The model under review builds one solid part; all positions refer to its coordinate system, in mm. A direction names the side the tool comes from. Round coordinates to 2 decimals unless told otherwise and drop trailing zeros. Order: outer loops, then holes, each group sorted by start corner. A loop starts at its lowest first (then second) coordinate and runs counter-clockwise, first axis right, second up. Notation, with made-up numbers: M 80,83 L 110,83 A26 ccw 110,108 Z; hole C 24,-17 d11. An arc over 180 degrees is marked long. Answer as a JSON object with one key per item and string values. Group by question number.
1) The part is to be moulded in two halves that separate along Y. For faces 3 (the flat face through (25.4, 0, 38)), 4 (the cylindrical face through (0.33, -2.52, 37.57)), 5 (the flat face through (2, -2, 0)), 6 (the cylindrical face through (-7.268, -2.289, 37.567)), say which applies: +Y half, -Y half, draft (parallel to the pull), parting line (faces both ways), or undercut.
2) Consider section A-A, the plane y = 0. Write out the cut boundary in (x, z).
3) Consider section C-C, the plane z = 29.5. Write out the cut boundary in (x, y) (3 decimals), then the cut area to 3 significant figures.
4) Consider section D-D, the plane x = 18. Write out the cut boundary in (y, z), then the cut area to 3 significant figures.
5) To check wall thickness, follow line 1 (Z direction, x = 44, y = 1.5); line 2 (Y direction, x = 0, z = 20); line 3 (Y direction, x = 28, z = 21) (3 decimals). State the ranges of each line that lie inside material, in increasing order.
6) Consider section B-B, the plane x = 41. Write out the cut boundary in (y, z) (3 decimals).
7) For faces 1 (the flat face through (38, 0, 57.15)), 2 (the flat face through (2, -2, 76.2)), list the 3-axis set-ups (+Z, -Z, +X, -X, +Y, -Y) from which the entire face can be reached by the end or side of a thin tool; tool diameter is ignored.
8) Insertion check: pin 1 Ø5 at (x, y) = (40, 0) entering from +Z; pin 2 Ø1.9 at (x, y) = (33.5, -1) entering from -Z. Each pin has a flat end and moves straight along its axis. Give the tip position at first contact, or say it passes through.
```python
from build123d import *

# Parameters (mm, degrees)
SKETCH4_R               = 7.62
SKETCH4_R_2             = 2.54
BOSS_EXTRUDE1_DEPTH     = 76.2
SKETCH5_W               = 63.5
SKETCH5_H               = 15.24
BOSS_EXTRUDE2_DEPTH     = 50.8
SKETCH6_W               = 38.1
SKETCH6_H               = 6.35
CUT_EXTRUDE1_DEPTH      = 25.4
CUT_EXTRUDE2_DEPTH      = 92.897466777
CUT_EXTRUDE2_DEPTH_BACK = 92.897466777
SKETCH7_R               = 2.54


with BuildPart() as part:
    # Sketch4 → Boss-Extrude1 (new body)
    with BuildSketch(Plane.XY):
        with Locations(Location((0, 0, 0), (0, 0, 180))):
            Circle(SKETCH4_R)
        with Locations(Location((0, 0, 0), (0, 0, 180))):
            Circle(SKETCH4_R_2, mode=Mode.SUBTRACT)
    extrude(amount=BOSS_EXTRUDE1_DEPTH)

    # Sketch5 → Boss-Extrude2 (add)
    with BuildSketch(Plane(origin=(0, 0, 0), x_dir=(0, 0, -1), z_dir=(1, 0, 0))):
        with Locations((-38.1, 0)):
            Rectangle(SKETCH5_W, SKETCH5_H)
    extrude(amount=BOSS_EXTRUDE2_DEPTH)

    # Sketch6 → Cut-Extrude1 (cut)
    with BuildSketch(Plane(origin=(50.8, 0, 0), x_dir=(0, 0, -1), z_dir=(1, 0, 0))):
        with Locations((-38.1, 0)):
            Rectangle(SKETCH6_W, SKETCH6_H)
    extrude(amount=-CUT_EXTRUDE1_DEPTH, mode=Mode.SUBTRACT)

    # Sketch7 → Cut-Extrude2 (cut, two sides: drawn at the far end of the back side and taken through both)
    with BuildSketch(Plane.XY.offset(-CUT_EXTRUDE2_DEPTH_BACK)):
        with Locations(Location((0, 0, 0), (0, 0, 180))):
            Circle(SKETCH7_R)
    extrude(amount=CUT_EXTRUDE2_DEPTH + CUT_EXTRUDE2_DEPTH_BACK, mode=Mode.SUBTRACT)


solid = part.part
```
Results list:
{
 "1": {"face 3": "undercut", "face 4": "undercut", "face 5": "draft", "face 6": "parting line"},
 "2": {"outline": "M -7.62,0 L -2.54,0 L -2.54,76.2 L -7.62,76.2 Z; M 2.54,0 L 7.62,0 L 7.62,6.35 L 50.8,6.35 L 50.8,19.05 L 25.4,19.05 L 25.4,57.15 L 50.8,57.15 L 50.8,69.85 L 7.62,69.85 L 7.62,76.2 L 2.54,76.2 Z"},
 "3": {"outline": "M 0,-7.62 L 50.8,-7.62 L 50.8,-3.175 L 25.4,-3.175 L 25.4,3.175 L 50.8,3.175 L 50.8,7.62 L 0,7.62 A7.62 ccw Z; hole C 0,0 d5.08", "area": "684 mm^2"},
 "4": {"outline": "M -7.62,6.35 L 7.62,6.35 L 7.62,69.85 L -7.62,69.85 Z", "area": "968 mm^2"},
 "5": {"line 1": "6.35 to 19.05, 57.15 to 69.85", "line 2": "-7.62 to -2.54, 2.54 to 7.62", "line 3": "-7.62 to -3.175, 3.175 to 7.62"},
 "6": {"outline": "M -7.62,6.35 L 7.62,6.35 L 7.62,69.85 L -7.62,69.85 Z; hole M -3.175,19.05 L 3.175,19.05 L 3.175,57.15 L -3.175,57.15 Z"},
 "7": {"face 1": "+X", "face 2": "+Z, +X, -X, +Y, -Y"},
 "8": {"pin 1": "z = 69.85", "pin 2": "z = 6.35"}
}
